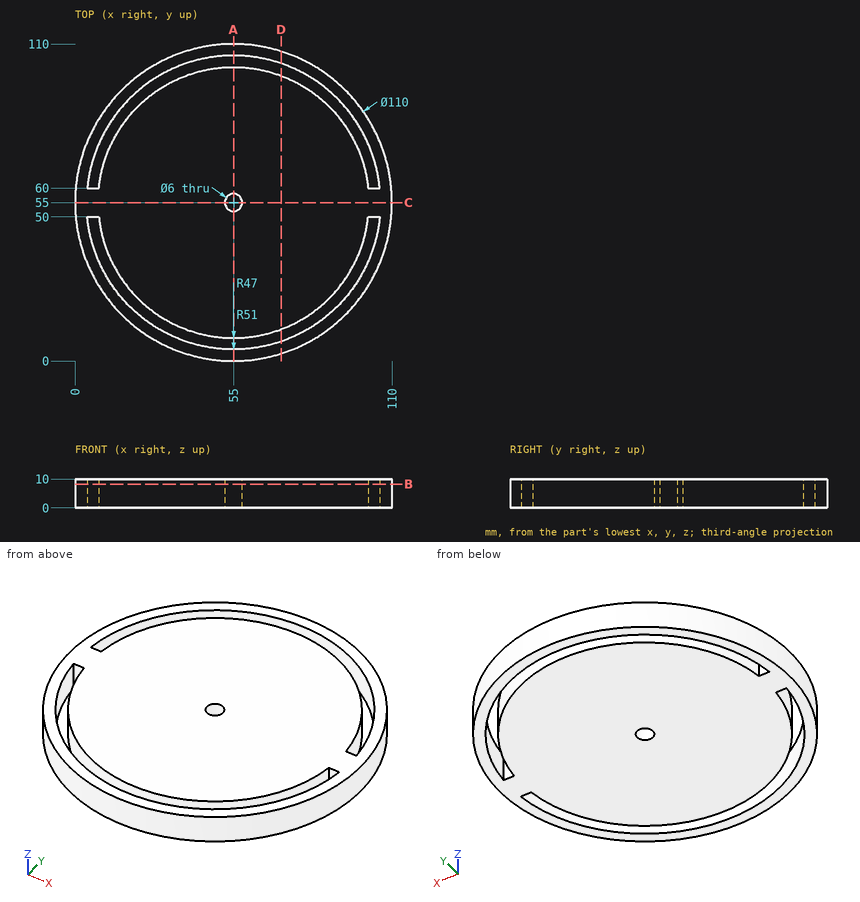
For this review, use the dimensioned drawing (mm, ordinates from the lowest corner) and the shaded views. Give positions to 0.01 mm unless a question says otherwise; leave off trailing zeros. Order: outer loops, then holes, each group sorted by start corner. A loop starts at its lowest first (then second) coordinate and runs counter-clockwise, first axis right, second up. Notation, with made-up numbers: (70, 15) - (107, 15) arc R34 cw to (107, 53) - close; hole circle Ø5 at (10.5, -20). An arc over 180 degrees is marked (long way). Write item = value, one per line. Start each with the question number.
Q1. We need section D-D on x = 71.5. State the section outline as (y, z) points, plus the area to 3 significant figures.
Q2. We need section C-C on y = 55. State the section outline as (x, z) points, plus the area to 3 significant figures.
Q3. We need section A-A on x = 55. State the section outline as (y, z) points, plus the area to 3 significant figures.
Q4. We need section B-B on z = 8.25. State the section outline as (x, y) points.
Q5. Clearance check with flat-ended pins moving along their axes: pin 1 Ø4.5 at (x, z) = (7, 5.5) entering from +Y; pin 2 Ø4.5 at (x, z) = (104, 3) entering from -Y; pin 3 Ø4 at (x, z) = (16.5, 5) entering from +Y. State where each tip first meets the part, or that it passes through.
Q6. To check wall thickness, follow L1, parallel to Y at x = 55, z = 6; L2, parallel to X at y = 48, z = 9.5; L3, parallel to Y at x = 41.5, z = 1.25. State the ranges of each line that lie inside material, in increasing order. Write a range as from..to.
Working result:
q1.outline = (2.53, 0) - (6.74, 0) - (6.74, 10) - (2.53, 10) - close; (10.99, 0) - (99.01, 0) - (99.01, 10) - (10.99, 10) - close; (103.26, 0) - (107.47, 0) - (107.47, 10) - (103.26, 10) - close
q1.area = 964 mm²
q2.outline = (0, 0) - (52, 0) - (52, 10) - (0, 10) - close; (58, 0) - (110, 0) - (110, 10) - (58, 10) - close
q2.area = 1,040 mm²
q3.outline = (0, 0) - (4, 0) - (4, 10) - (0, 10) - close; (8, 0) - (52, 0) - (52, 10) - (8, 10) - close; (58, 0) - (102, 0) - (102, 10) - (58, 10) - close; (106, 0) - (110, 0) - (110, 10) - (106, 10) - close
q3.area = 960 mm²
q4.outline = circle Ø110 at (55, 55); hole (4.25, 50) arc R51 ccw to (105.75, 50) - (101.73, 50) arc R47 cw to (8.27, 50) - close; hole (4.25, 60) - (8.27, 60) arc R47 cw to (101.73, 60) - (105.75, 60) arc R51 ccw to start; hole circle Ø6 at (55, 55)
q5.pin_1 = 85.53
q5.pin_2 = 26.03
q5.pin_3 = 96.14
q6.L1 = 0..4, 8..52, 58..102, 106..110
q6.L2 = 0.45..4.48, 8.52..101.48, 105.52..109.55
q6.L3 = 1.68..5.82, 9.98..100.02, 104.18..108.32
